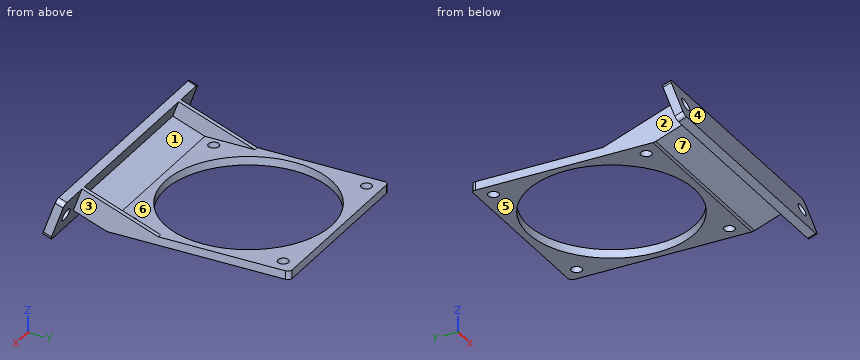
Autodesk Inventor part; units mm, degrees
ref_plane "YZ Plane" through (0, 0, 0) normal (1, 0, 0) x (0, 1, 0)
ref_plane "XZ Plane" through (0, 0, 0) normal (0, 1, 0) x (-1, 0, 0)
ref_plane "XY Plane" through (0, 0, 0) normal (0, 0, 1) x (1, 0, 0)
sketch "Sketch1" plane through (0, 0, 0) normal (0, 0, 1) x (1, 0, 0)
  line L0 (-35.75, 35.75) -> (35.75, -35.75) construction
  line L1 (35.75, 35.75) -> (-35.75, -35.75) construction
  line L2 (-42.5, 42.5) -> (42.5, 42.5)
  line L3 (42.5, 42.5) -> (42.5, -42.5)
  line L4 (42.5, -42.5) -> (-42.5, -42.5)
  line L5 (-42.5, -42.5) -> (-42.5, 42.5)
  line L6 (-42.5, 42.5) -> (42.5, -42.5) construction
  line L7 (42.5, 42.5) -> (-42.5, -42.5) construction
  circle A0 centre (-35.75, 35.75) radius 2.5
  circle A1 centre (35.75, 35.75) radius 2.5
  circle A2 centre (-35.75, -35.75) radius 2.5
  circle A3 centre (35.75, -35.75) radius 2.5
  circle A4 centre (0, 0) radius 39
  dimension "d0" = 71.5
  dimension "d1" = 71.5
  dimension "d2" = 85
  dimension "d3" = 85
  dimension "d4" = 5
  dimension "d5" = 5
  dimension "d6" = 5
  dimension "d7" = 5
  dimension "d8" = 78
extrude "Extrusion1" add sketch "Sketch1" along normal blind 4
ref_plane "Work Plane2" through (42.5, -42.5, 4) normal (0, -0.342, -0.9397) x (1, 0, 0)
sketch "Sketch4" plane through (42.5, -42.5, 4) normal (0, -0.342, -0.9397) x (1, 0, 0)
  line L0 (-85, 0) -> (0, 0)
  line L1 (0, 0) -> (-85, 0)
  line L2 (-85, 0) -> (-85, 16)
  line L3 (-85, 16) -> (0, 16)
  line L4 (0, 16) -> (0, 0)
  point P0 (-42.5, -41.305)
  dimension "d15" = 16
extrude "Extrusion2" add sketch "Sketch4" along normal blind 4
sketch "Sketch5" plane through (42.5, -57.5351, 9.4723) normal (1, 0, 0) x (0, -0.342, -0.9397)
  line L0 (0, 0) -> (0, 16)
  line L1 (3.7588, 17.3681) -> (0, 16)
  line L2 (0, 16) -> (3.7588, 17.3681)
  line L3 (4, 16) -> (4, 0)
  line L4 (3.7588, 17.3681) -> (4, 16)
  line L5 (4, 16) -> (0, 16)
  point P0 (-10.7771, 57.305)
extrude "Extrusion3" add sketch "Sketch5" against normal blind 85
sketch "Sketch6" plane through (-42.5, -57.5351, 9.4723) normal (0, -0.9397, 0.342) x (1, 0, 0)
  line L0 (85, 0) -> (85, -4)
  line L1 (85, -4) -> (0, 0)
  line L2 (100, -12) -> (-15, -12)
  line L3 (-15, -12) -> (-15, 8)
  line L4 (-15, 8) -> (100, 8)
  line L5 (100, 8) -> (100, -12)
  line L6 (100, -12) -> (-15, 8) construction
  line L7 (-15, -12) -> (100, 8) construction
  circle A0 centre (92.5, -2) radius 3
  line L8 (42.5, 8) -> (42.5, -12)
  circle A1 centre (-7.5, -2) radius 3
  point P0 (42.5, -2)
  dimension "d20" = 115
  dimension "d21" = 20
  dimension "d22" = 6
  dimension "d23" = 7.5
extrude "Extrusion4" add sketch "Sketch6" along normal blind 4
fillet "Fillet1" radius 2 6 edges at (57.5, -63.5187, -1.1199) (-57.5, -63.5187, -1.1199) (-57.5, -56.6783, 17.6739) (57.5, -56.6783, 17.6739) (42.5, 42.5, 2) (-42.5, 42.5, 2)
sketch "Sketch8" plane through (-42.5, -57.5351, 9.4723) normal (0, 0.9397, -0.342) x (1, 0, 0)
  line L0 (0, 0) -> (2, 0)
  line L1 (2, 0) -> (2, -8)
  line L2 (2, -8) -> (0, -8)
  line L3 (0, -8) -> (0, 0)
  point P0 (42.5, -10.7771)
  dimension "d33" = 2
  dimension "d34" = 8
extrude "Extrusion6" add sketch "Sketch8" along normal up to surface surface through (0, 0, 4) normal (0, 0, 1)
ref_plane "Work Plane3" through (0, -42.5, 0) normal (-1, 0, 0) x (0, 0, 1)
mirror "Mirror1" about plane through (0, -42.5, 0) normal (-1, 0, 0) of "Extrusion6"
properties part number "Eletronica - FanPlaca"
Can you work these out from the model? Positions are in its coordinate system, mm. Face numbers are marked on the shaded views. A direction names the side the tool comes from. Coordinates: 2 decimals unless noted, no trailing zeros. Order: outer loops, then holes, each group sorted by start corner. A loop starts at its lowest first (then second) coordinate and runs counter-clockwise, first axis right, second up. Notation, with made-up numbers: M 31,-20 L 71,-20 A14 ccw 71,-16 Z; hole C 79,-26.5 d7. An arc over 180 degrees is marked long. Answer as CSV lines item,"result".
(1) Please list where these lines run through material, in increasing order: L1, parallel to X at y = -30, z = 5.25; L2, parallel to X at y = -56.5, z = 8.5; L3, parallel to Z at x = 39, y = 16.
Geometry check:
L1,"-42.5 to -40.5, 40.5 to 42.5"
L2,"-42.5 to 42.5"
L3,"0 to 4"
(2) Suppose I cut it at C-C on y = 20.5. Please give me the cut outline in (x, z).
Geometry check:
outline,"M -42.5,0 L -33.18,0 L -33.18,4 L -42.5,4 Z; M 33.18,0 L 42.5,0 L 42.5,4 L 33.18,4 Z"
(3) If we mould it in two halves opening along X, with no side actions, what happens to the marked faces 1, 2 and 3? For each: released by +X, released by -X, zero draft, split by the parting line, or undercut.
Geometry check:
face 1,"undercut"
face 2,"released by -X"
face 3,"released by +X"
(4) Suppose I cut it at B-B on y = -35.75. Please give me the cut outline in (x, z), plus the area to 3 significant figures.
Geometry check:
outline,"M -42.5,0 L -38.25,0 L -38.25,4 L -40.5,4 L -40.5,10.06 L -42.5,10.06 Z; M -33.25,0 L -15.59,0 L -15.59,4 L -33.25,4 Z; M 15.59,0 L 33.25,0 L 33.25,4 L 15.59,4 Z; M 38.25,0 L 42.5,0 L 42.5,10.06 L 40.5,10.06 L 40.5,4 L 38.25,4 Z"
area,"200 mm^2"
(5) I'm going to push flat-ended pins straight in: pin 1 (4 mm diameter, centred on x = -35.75, y = 35.75, fed in from -Z); pin 2 (8 mm diameter, centred on x = 34.5, y = -40.5, fed in from -Z); pin 3 (4 mm diameter, centred on x = -35, y = 16.5, fed in from +Z); pin 4 (6.5 mm diameter, centred on y = -43, z = 10, fed in from +X). Where does each tip first touch, or does it pass through?
Geometry check:
pin 1,"through"
pin 2,"z = 0"
pin 3,"z = 4"
pin 4,"x = 42.5"
(6) Suppose I cut it at A-A on x = 35.75. Count the separate pieces of the cut face and the enclosed holes in it, plus the area to 3 significant figures.
Geometry check:
separate pieces,"4"
enclosed holes,"0"
area,"322 mm^2"
(7) On a 3-axis mill with a long thin cutter (end or side, diameter ignored), from which of +Z, -Z, +X, -X, +Y, -Y can I reach the whole of each face in a straight line? I mean the marked faces 4, 5, 6 and 7. Say none if no direction works.
Geometry check:
face 4,"+Z, +X, -X, -Y"
face 5,"-Z, +X, -X, +Y"
face 6,"+Z, +Y"
face 7,"-Z, +X, -X"
